from build123d import *

# Parameters (mm, degrees)
SKETCH1_W               = 20
SKETCH1_H               = 63.5
BOSS_EXTRUDE1_DEPTH     = 12.7
SKETCH2_R               = 3.175
SKETCH2_R_2             = 2.1844
CUT_EXTRUDE1_DEPTH      = 36.62797356
CUT_EXTRUDE2_DEPTH      = 36.62797356
CUT_EXTRUDE2_DEPTH_BACK = 36.62797356
SKETCH4_R               = 3.81
CUT_EXTRUDE3_DEPTH      = 8.89
SKETCH4_3_R             = 3.81
SKETCH4_3_R_2           = 2.1844
SKETCH4_3_R_3           = 5.334
SKETCH4_3_R_4           = 3.175
CUT_EXTRUDE4_DEPTH      = 3.81
CUT_EXTRUDE5_REACH      = 36.454
SKETCH6_R               = 5.08
SKETCH6_R_2             = 2.667
CUT_EXTRUDE6_DEPTH      = 10
CUT_EXTRUDE6_DEPTH_BACK = 35.454239272
SKETCH6_4_R             = 2.159
SKETCH6_4_R_2           = 2.667
FILLET1_R               = 10.16


with BuildPart() as part:
    # Sketch1 → Boss-Extrude1 (new body)
    with BuildSketch(Plane(origin=(0, 0, 0), x_dir=(1, 0, 0), z_dir=(0, 1, 0))):
        Rectangle(SKETCH1_W, SKETCH1_H)
    extrude(amount=BOSS_EXTRUDE1_DEPTH)

    # Sketch2 → Cut-Extrude1 (cut, through all)
    with BuildSketch(Plane(origin=(0, 12.7, 0), x_dir=(1, 0, 0), z_dir=(0, 1, 0))):
        with Locations(Location((0, 0, 0), (0, 0, 270))):
            Circle(SKETCH2_R)
        with Locations(Location((-4.912200098, 4.912200098, 0), (0, 0, 270))):
            Circle(SKETCH2_R_2)
        with Locations(Location((4.912200098, -4.912200098, 0), (0, 0, 270))):
            Circle(SKETCH2_R_2)
        with Locations(Location((4.912200098, 4.912200098, 0), (0, 0, 90))):
            Circle(SKETCH2_R_2)
        with Locations(Location((-4.912200098, -4.912200098, 0), (0, 0, 90))):
            Circle(SKETCH2_R_2)
    extrude(amount=-CUT_EXTRUDE1_DEPTH, mode=Mode.SUBTRACT)

    # Sketch3 → Cut-Extrude2 (cut, two sides: drawn at the far end of the back side and taken through both)
    with BuildSketch(Plane(origin=(0, 0, 0), x_dir=(0, 0, -1), z_dir=(1, 0, 0)).offset(-CUT_EXTRUDE2_DEPTH_BACK)):
        with BuildLine():
            Line((31.75, 3.81), (31.75, 12.7))
            Line((31.75, 12.7), (10.906600098, 12.7))
            ThreePointArc((10.906600098, 12.7), (16.898665682, 6.209564949), (25.4, 3.81))
            Line((25.4, 3.81), (31.75, 3.81))
        make_face()
        with BuildLine():
            ThreePointArc((-25.4, 3.81), (-16.898665682, 6.209564949), (-10.906600098, 12.7))
            Line((-10.906600098, 12.7), (-31.75, 12.7))
            Line((-31.75, 12.7), (-31.75, 3.81))
            Line((-31.75, 3.81), (-25.4, 3.81))
        make_face()
    extrude(amount=CUT_EXTRUDE2_DEPTH + CUT_EXTRUDE2_DEPTH_BACK, mode=Mode.SUBTRACT)

    # Sketch4 → Cut-Extrude3 (cut)
    with BuildSketch(Plane.XZ):
        with Locations((-4.912200098, -4.912200098)):
            Circle(SKETCH4_R)
        with Locations((4.912200098, 4.912200098)):
            Circle(SKETCH4_R)
        with Locations((-4.912200098, 4.912200098)):
            Circle(SKETCH4_R)
        with Locations((4.912200098, -4.912200098)):
            Circle(SKETCH4_R)
    extrude(amount=-CUT_EXTRUDE3_DEPTH, mode=Mode.SUBTRACT)

    # Sketch4<3> → Cut-Extrude4 (cut)
    # profile 1 of 28: a face of its own
    with BuildSketch(Plane.XZ):
        with Locations((-4.912200098, 4.912200098)):
            Circle(SKETCH4_3_R)
        with Locations(Location((-4.912200098, 4.912200098, 0), (0, 0, 270))):
            Circle(SKETCH4_3_R_2, mode=Mode.SUBTRACT)
    # profile 2 of 28: a face of its own
    with BuildSketch(Plane.XZ):
        Circle(SKETCH4_3_R_3)
        with Locations(Location((0, 0, 0), (0, 0, 90))):
            Circle(SKETCH4_3_R_4, mode=Mode.SUBTRACT)
    # profile 3 of 28: a face of its own
    with BuildSketch(Plane.XZ):
        Circle(SKETCH4_3_R_3)
    # profile 4 of 28: a face of its own
    with BuildSketch(Plane.XZ):
        with Locations(Location((-4.912200098, 4.912200098, 0), (0, 0, 270))):
            Circle(SKETCH4_3_R_2)
    # profile 5 of 28: a face of its own
    with BuildSketch(Plane.XZ):
        with Locations((-4.912200098, 4.912200098)):
            Circle(SKETCH4_3_R)
    # profile 6 of 28: a face of its own
    with BuildSketch(Plane.XZ):
        Circle(SKETCH4_3_R_3)
        with Locations(Location((0, 0, 0), (0, 0, 90))):
            Circle(SKETCH4_3_R_4, mode=Mode.SUBTRACT)
    # profile 7 of 28: a face of its own
    with BuildSketch(Plane.XZ):
        with Locations((-4.912200098, -4.912200098)):
            Circle(SKETCH4_3_R)
    # profile 8 of 28: a face of its own
    with BuildSketch(Plane.XZ):
        Circle(SKETCH4_3_R_3)
        with Locations(Location((0, 0, 0), (0, 0, 90))):
            Circle(SKETCH4_3_R_4, mode=Mode.SUBTRACT)
    # profile 9 of 28: a face of its own
    with BuildSketch(Plane.XZ):
        with Locations((-4.912200098, -4.912200098)):
            Circle(SKETCH4_3_R)
        with Locations(Location((-4.912200098, -4.912200098, 0), (0, 0, 90))):
            Circle(SKETCH4_3_R_2, mode=Mode.SUBTRACT)
    # profile 10 of 28: a face of its own
    with BuildSketch(Plane.XZ):
        Circle(SKETCH4_3_R_3)
    # profile 11 of 28: a face of its own
    with BuildSketch(Plane.XZ):
        with Locations(Location((-4.912200098, -4.912200098, 0), (0, 0, 90))):
            Circle(SKETCH4_3_R_2)
    # profile 12 of 28: a face of its own
    with BuildSketch(Plane.XZ):
        with BuildLine():
            ThreePointArc((1.973854475, -2.486870224), (1.04518229, -2.998035854), (0, -3.175))
            Line((0, -3.175), (0, -5.334))
            ThreePointArc((0, -5.334), (0.560277089, -5.304492962), (1.114355409, -5.216298306))
            ThreePointArc((1.114355409, -5.216298306), (1.278123958, -3.767826643), (1.973854475, -2.486870224))
        make_face()
    # profile 13 of 28: a face of its own
    with BuildSketch(Plane.XZ):
        with BuildLine():
            Line((0, -5.334), (0, -3.175))
            ThreePointArc((0, -3.175), (-1.04518229, -2.998035854), (-1.973854475, -2.486870224))
            ThreePointArc((-1.973854475, -2.486870224), (-1.326729639, -3.623595587), (-1.102200098, -4.912200098))
            ThreePointArc((-1.102200098, -4.912200098), (-1.105240139, -5.064370621), (-1.114355409, -5.216298306))
            ThreePointArc((-1.114355409, -5.216298306), (-0.560277089, -5.304492962), (0, -5.334))
        make_face()
    # profile 14 of 28: a face of its own
    with BuildSketch(Plane.XZ):
        with Locations((4.912200098, -4.912200098)):
            Circle(SKETCH4_3_R)
        with Locations(Location((4.912200098, -4.912200098, 0), (0, 0, 270))):
            Circle(SKETCH4_3_R_2, mode=Mode.SUBTRACT)
    # profile 15 of 28: a face of its own
    with BuildSketch(Plane.XZ):
        Circle(SKETCH4_3_R_3)
        with Locations(Location((0, 0, 0), (0, 0, 90))):
            Circle(SKETCH4_3_R_4, mode=Mode.SUBTRACT)
    # profile 16 of 28: a face of its own
    with BuildSketch(Plane.XZ):
        Circle(SKETCH4_3_R_3)
    # profile 17 of 28: a face of its own
    with BuildSketch(Plane.XZ):
        with Locations(Location((4.912200098, -4.912200098, 0), (0, 0, 270))):
            Circle(SKETCH4_3_R_2)
    # profile 18 of 28: a face of its own
    with BuildSketch(Plane.XZ):
        with Locations((4.912200098, -4.912200098)):
            Circle(SKETCH4_3_R)
    # profile 19 of 28: a face of its own
    with BuildSketch(Plane.XZ):
        Circle(SKETCH4_3_R_3)
        with Locations(Location((0, 0, 0), (0, 0, 90))):
            Circle(SKETCH4_3_R_4, mode=Mode.SUBTRACT)
    # profile 20 of 28: a face of its own
    with BuildSketch(Plane.XZ):
        with Locations((4.912200098, 4.912200098)):
            Circle(SKETCH4_3_R)
    # profile 21 of 28: a face of its own
    with BuildSketch(Plane.XZ):
        Circle(SKETCH4_3_R_3)
        with Locations(Location((0, 0, 0), (0, 0, 90))):
            Circle(SKETCH4_3_R_4, mode=Mode.SUBTRACT)
    # profile 22 of 28: a face of its own
    with BuildSketch(Plane.XZ):
        with Locations((4.912200098, 4.912200098)):
            Circle(SKETCH4_3_R)
        with Locations(Location((4.912200098, 4.912200098, 0), (0, 0, 90))):
            Circle(SKETCH4_3_R_2, mode=Mode.SUBTRACT)
    # profile 23 of 28: a face of its own
    with BuildSketch(Plane.XZ):
        Circle(SKETCH4_3_R_3)
    # profile 24 of 28: a face of its own
    with BuildSketch(Plane.XZ):
        with Locations(Location((4.912200098, 4.912200098, 0), (0, 0, 90))):
            Circle(SKETCH4_3_R_2)
    # profile 25 of 28: a face of its own
    with BuildSketch(Plane.XZ):
        with BuildLine():
            Line((0, 3.175), (0, 5.334))
            ThreePointArc((0, 5.334), (-0.560277089, 5.304492962), (-1.114355409, 5.216298306))
            ThreePointArc((-1.114355409, 5.216298306), (-1.105240139, 5.064370621), (-1.102200098, 4.912200098))
            ThreePointArc((-1.102200098, 4.912200098), (-1.326729639, 3.623595587), (-1.973854475, 2.486870224))
            ThreePointArc((-1.973854475, 2.486870224), (-1.04518229, 2.998035854), (0, 3.175))
        make_face()
    # profile 26 of 28: a face of its own
    with BuildSketch(Plane.XZ):
        with BuildLine():
            ThreePointArc((1.114355409, 5.216298306), (0.560277089, 5.304492962), (0, 5.334))
            Line((0, 5.334), (0, 3.175))
            ThreePointArc((0, 3.175), (1.04518229, 2.998035854), (1.973854475, 2.486870224))
            ThreePointArc((1.973854475, 2.486870224), (1.278123958, 3.767826643), (1.114355409, 5.216298306))
        make_face()
    # profile 27 of 28: a face of its own
    with BuildSketch(Plane.XZ):
        with BuildLine():
            ThreePointArc((1.973854475, 2.486870224), (1.04518229, 2.998035854), (0, 3.175))
            Line((0, 3.175), (0, -3.175))
            ThreePointArc((0, -3.175), (1.04518229, -2.998035854), (1.973854475, -2.486870224))
            ThreePointArc((1.973854475, -2.486870224), (2.218123262, -2.218123262), (2.486870224, -1.973854475))
            ThreePointArc((2.486870224, -1.973854475), (2.998035854, -1.04518229), (3.175, 0))
            ThreePointArc((3.175, 0), (2.998035854, 1.04518229), (2.486870224, 1.973854475))
            ThreePointArc((2.486870224, 1.973854475), (2.218123262, 2.218123262), (1.973854475, 2.486870224))
        make_face()
    # profile 28 of 28: a face of its own
    with BuildSketch(Plane.XZ):
        with BuildLine():
            Line((0, -3.175), (0, 3.175))
            ThreePointArc((0, 3.175), (-1.04518229, 2.998035854), (-1.973854475, 2.486870224))
            ThreePointArc((-1.973854475, 2.486870224), (-2.218123262, 2.218123262), (-2.486870224, 1.973854475))
            ThreePointArc((-2.486870224, 1.973854475), (-3.175, 0), (-2.486870224, -1.973854475))
            ThreePointArc((-2.486870224, -1.973854475), (-2.218123262, -2.218123262), (-1.973854475, -2.486870224))
            ThreePointArc((-1.973854475, -2.486870224), (-1.04518229, -2.998035854), (0, -3.175))
        make_face()
    extrude(amount=-CUT_EXTRUDE4_DEPTH, mode=Mode.SUBTRACT)

    # Cut-Extrude5: up to this face of the body (flat: up to its plane)
    cut_extrude5_end = Plane(part.part.faces().sort_by_distance((9.704058164, 12.7, 0))[0])
    # Sketch6 → Cut-Extrude5 (cut, up to the picked face)
    with BuildSketch(Plane(origin=(0, 3.81, 0), x_dir=(1, 0, 0), z_dir=(0, 1, 0)), mode=Mode.PRIVATE) as cut_extrude5_sk1:
        with Locations(Location((0, 19.812, 0), (0, 0, 90))):
            Circle(SKETCH6_R)
    cut_extrude5_tool1 = split(extrude(cut_extrude5_sk1.sketch, amount=CUT_EXTRUDE5_REACH, mode=Mode.PRIVATE), bisect_by=cut_extrude5_end, keep=Keep.BOTH, mode=Mode.PRIVATE)
    # Sketch6 → Cut-Extrude5 (cut, up to the picked face)
    with BuildSketch(Plane(origin=(0, 3.81, 0), x_dir=(1, 0, 0), z_dir=(0, 1, 0)), mode=Mode.PRIVATE) as cut_extrude5_sk2:
        with Locations(Location((0, -19.812, 0), (0, 0, 90))):
            Circle(SKETCH6_R)
        with Locations(Location((0, -19.812, 0), (0, 0, 90))):
            Circle(SKETCH6_R_2, mode=Mode.SUBTRACT)
    cut_extrude5_tool2 = split(extrude(cut_extrude5_sk2.sketch, amount=CUT_EXTRUDE5_REACH, mode=Mode.PRIVATE), bisect_by=cut_extrude5_end, keep=Keep.BOTH, mode=Mode.PRIVATE)
    add(cut_extrude5_tool1.solids().sort_by(Axis((0, 3.81, -19.812), (0, 1, 0)))[0], mode=Mode.SUBTRACT)
    add(cut_extrude5_tool2.solids().sort_by(Axis((0, 3.81, 24.748316), (0, 1, 0)))[0], mode=Mode.SUBTRACT)

    # Sketch6<4> → Cut-Extrude6 (cut, two sides: drawn at the far end of the back side and taken through both)
    with BuildSketch(Plane(origin=(0, 3.81, 0), x_dir=(1, 0, 0), z_dir=(0, 1, 0)).offset(-CUT_EXTRUDE6_DEPTH_BACK)):
        with Locations((0, 19.812)):
            Circle(SKETCH6_4_R)
        with Locations((0, -19.812)):
            Circle(SKETCH6_4_R)
        with Locations(Location((0, 19.812, 0), (0, 0, 270))):
            Circle(SKETCH6_4_R_2)
        with Locations(Location((0, -19.812, 0), (0, 0, 270))):
            Circle(SKETCH6_4_R_2)
    extrude(amount=CUT_EXTRUDE6_DEPTH + CUT_EXTRUDE6_DEPTH_BACK, mode=Mode.SUBTRACT)

    # Fillet1
    # the kernel refuses this fillet: 10.16 mm, written as the material it takes off along each edge
    with BuildSketch(Plane(origin=(10, -25.4, 31.75), x_dir=(0, 0, -1), z_dir=(0, 1, 0)), Plane(origin=(10, -25.4, -31.75), x_dir=(-1, 0, 0), z_dir=(0, 1, 0)), Plane(origin=(-10, -25.4, 31.75), x_dir=(1, 0, 0), z_dir=(0, 1, 0))) as fillet1_piece_1:
        with BuildLine():
            CenterArc((FILLET1_R, FILLET1_R), FILLET1_R, 180, 90)
            Line((0, FILLET1_R), (0, 0))
            Line((0, 0), (FILLET1_R, 0))
        make_face()
    extrude(amount=54.61, mode=Mode.SUBTRACT)
    with BuildSketch(Plane(origin=(-10, -25.4, -31.75), x_dir=(1, 0, 0), z_dir=(0, 1, 0))) as fillet1_piece_2:
        with BuildLine():
            CenterArc((FILLET1_R, -FILLET1_R), FILLET1_R, 90, 90)
            Line((0, -FILLET1_R), (0, 0))
            Line((0, 0), (FILLET1_R, 0))
        make_face()
    extrude(amount=54.61, mode=Mode.SUBTRACT)


solid = part.part
The model under review builds one solid part; all positions refer to its coordinate system, in mm. A direction names the side the tool comes from. Coordinates: 2 decimals unless noted, no trailing zeros. Loops run counter-clockwise (first coordinate to the right, second up) from the corner with the lowest first, then second, coordinate; pieces in that order, holes last.
(1) Tool access review of faces 5 (the cylindrical face through (-0.14, 8.591, 13.884)), 6 (the cylindrical face through (-7.72, 4.38, -7.49)), 7 (the flat face through (2, 3.81, -22)): name each direction out of +Z, -Z, +X, -X, +Y, -Y from which nothing blocks a thin tool from reaching the whole face with its end or side.
Determined:
face 5: +Z, +X, -X, +Y
face 6: -Y
face 7: +Y
(2) Consider section D-D, the plane z = 14. Give the boundary of the cut face in (x, y), plus the area to 3 significant figures.
Determined:
outline: (-10, 0) - (10, 0) - (10, 8.48) - (-10, 8.48) - close
area: 170 mm2
(3) Draft analysis for pull direction Z (two halves, no side actions). For faces 1 (the cylindrical face through (7.158, 2.102, -28.638)), 2 (the flat face through (0, 3.81, 28)), 3 (the cylindrical face through (-1.22, 8.32, 2.93)), 4 (the cylindrical face through (-7.045, 10.822, -5.386)), state which applies: +Z half, -Z half, draft (parallel to the pull), parting line (faces both ways), or undercut.
Determined:
face 1: -Z half
face 2: draft
face 3: undercut
face 4: undercut
(4) Consider section A-A, the plane z = 0. Give the boundary of the cut face in (x, y) (3 decimals), plus the area to 3 significant figures.
Determined:
outline: (-10, 0) - (-5.334, 0) - (-5.334, 3.81) - (-3.175, 3.81) - (-3.175, 12.7) - (-10, 12.7) - close; (3.175, 3.81) - (5.334, 3.81) - (5.334, 0) - (10, 0) - (10, 12.7) - (3.175, 12.7) - close
area: 157 mm2
(5) Consider section C-C, the plane z = -18. Give the boundary of the cut face in (x, y).
Determined:
outline: (-10, 0) - (-1.96, 0) - (-1.96, 3.81) - (-4.75, 3.81) - (-4.75, 5.59) - (-10, 5.59) - close; (1.96, 0) - (10, 0) - (10, 5.59) - (4.75, 5.59) - (4.75, 3.81) - (1.96, 3.81) - close
(6) Insertion check: P1, Ø3, axis at x = 3.5, z = 27.5, coming from the +Y side; P2, Ø4, axis at x = -1, y = 6.5, coming from the +Z side; P3, Ø2.5, axis at x = -4.91, z = -4.91, coming from the +Y side; P4, Ø6, axis at x = -2.5, y = 8.5, coming from the +Z side. Each pin has a flat end and moves straight along its axis. Give the tip position at first contact, or say it passes through.
Determined:
P1: stops at y = 3.81
P2: stops at z = 15.71
P3: passes through
P4: stops at z = 17.09
(7) Consider section B-B, the plane y = 5.5. Give the boundary of the cut face in (x, z) (3 decimals).
Determined:
outline: (-10, -18.182) - (-4.811, -18.182) arc R5.08 cw to (4.811, -18.182) - (10, -18.182) - (10, 18.182) - (4.811, 18.182) arc R5.08 cw to (-4.811, 18.182) - (-10, 18.182) - close; hole (-2.487, -1.974) arc R3.81 ccw (long way) to (-1.974, -2.487) arc R3.175 ccw to (1.974, -2.487) arc R3.81 ccw (long way) to (2.487, -1.974) arc R3.175 ccw to (2.487, 1.974) arc R3.81 ccw (long way) to (1.974, 2.487) arc R3.175 ccw to (-1.974, 2.487) arc R3.81 ccw (long way) to (-2.487, 1.974) arc R3.175 ccw to start
(8) Wall thickness on L1, parallel to Z at x = 6.5, y = 11.75; L2, parallel to X at y = 12.25, z = 0 (3 decimals); L3, parallel to Z at x = 5.75, y = 9.75: over which ranges is each line inside the solid? List them lowest first.
Determined:
L1: z = -11.43 to -6.41, -3.41 to 3.41, 6.41 to 11.43
L2: x = -10 to -3.175, 3.175 to 10
L3: z = -12.84 to -6.93, -2.89 to 2.89, 6.93 to 12.84
